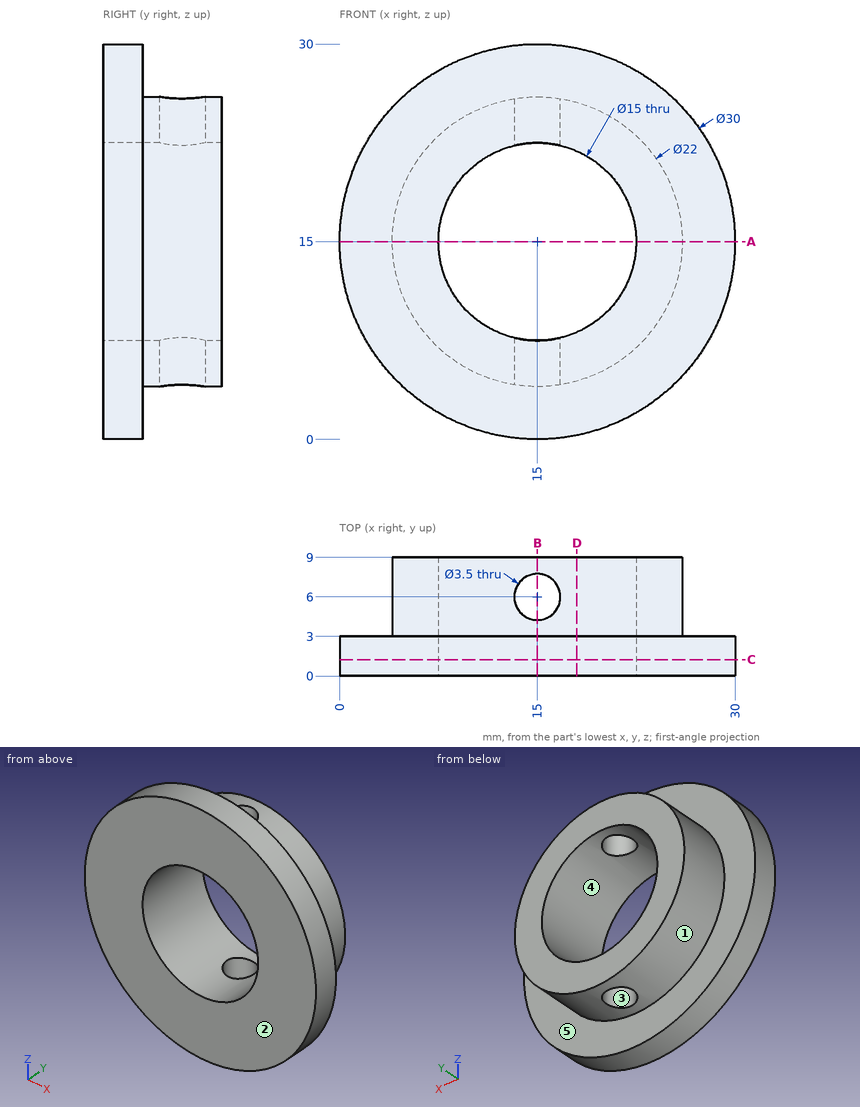
Part print with two shaded views. Sizes in mm from the minimum x, y, z corner. A direction names the side the tool comes from. Give positions to 0.01 mm unless a question says otherwise; leave off trailing zeros. Order: outer loops, then holes, each group sorted by start corner. A loop starts at its lowest first (then second) coordinate and runs counter-clockwise, first axis right, second up.
1) Wall check: probe 1 along X at (y, z) = (3.75, 15); probe 2 along X at (y, z) = (5, 13.25); probe 3 along Y at (x, z) = (8.5, 28). Give the ranges that are in metal, low to high.
2) Saw through at D-D, the plane x = 18. Write the cut outline in (y, z).
3) Mould opens along X. For the marked faces 1, 2 and 3 say: +X half, -X half, draft (parallel to the pull), parting line (faces both ways), or undercut.
4) Saw through at A-A, the plane z = 15. Write the cut outline in (x, y).
5) Saw through at B-B, the plane x = 15. Write the cut outline in (y, z).
6) Saw through at C-C, the plane y = 1.25. Write the cut outline in (x, z), then the cut area to 3 significant figures.
7) Pin check, flat tips, straight feed: pin 1 (2 mm diameter, centred on x = 16.5, y = 6.5, fed in from +Z); pin 2 (1 mm diameter, centred on y = 2, z = 20, fed in from -X); pin 3 (4.5 mm diameter, centred on x = 15, y = 6, fed in from -Z). Stop position of each tip, or through.
8) 3-axis set-ups, long thin cutter, end or side, ignore diameter. For the marked faces 4 and 5: which of +Z, -Z, +X, -X, +Y, -Y reach the whole face in a straight line?
Computed:
1. probe 1: x = 4 to 7.5, 22.5 to 26
1. probe 2: x = 4.14 to 7.71, 22.29 to 25.86
1. probe 3: y = 0 to 3
2. outline: (0, 0.3) - (3, 0.3) - (3, 4.42) - (9, 4.42) - (9, 8.13) - (0, 8.13) - close; (0, 21.87) - (9, 21.87) - (9, 25.58) - (3, 25.58) - (3, 29.7) - (0, 29.7) - close
3. face 1: parting line
3. face 2: draft
3. face 3: undercut
4. outline: (0, 0) - (7.5, 0) - (7.5, 9) - (4, 9) - (4, 3) - (0, 3) - close; (22.5, 0) - (30, 0) - (30, 3) - (26, 3) - (26, 9) - (22.5, 9) - close
5. outline: (0, 0) - (3, 0) - (3, 4) - (4.25, 4) - (4.25, 7.5) - (0, 7.5) - close; (0, 22.5) - (4.25, 22.5) - (4.25, 26) - (3, 26) - (3, 30) - (0, 30) - close; (7.75, 4) - (9, 4) - (9, 7.5) - (7.75, 7.5) - close; (7.75, 22.5) - (9, 22.5) - (9, 26) - (7.75, 26) - close
6. outline: circle Ø30 at (15, 15); hole circle Ø15 at (15, 15)
6. area: 530 mm2
7. pin 1: stops at z = 25.95
7. pin 2: stops at x = 0.69
7. pin 3: stops at z = 4
8. face 4: +Y, -Y
8. face 5: +Y
